Verification items for the finished model (mm, model axes). Give positions to 0.01 mm unless a question says otherwise; leave off trailing zeros. Order: outer loops, then holes, each group sorted by start corner. A loop starts at its lowest first (then second) coordinate and runs counter-clockwise, first axis right, second up. Notation, with made-up numbers: (-21, 55.25) - (17, 55.25) arc R28 ccw to (17, 78.25) - close; hole circle Ø3 at (-23.5, 14). An arc over 180 degrees is marked (long way). Answer as a JSON object with one key per item and string values. Group by question number.
(1) Mould release check, pull along Z, two halves, no side actions. Record for faces 1 (the face through (2, 7, 34.546)), 2 (the face through (-1.596, 6.902, -5.915)), 3 (the face through (2, 0, -1)), 4 (the face through (2, 7, -36.182)): +Z half, -Z half, draft (parallel to the pull), parting line (faces both ways), or undercut.
(2) Section check B-B (x = 3). Record the boundary of the cut face in (y, z).
(3) Section check C-C (y = 7). Record the boundary of the cut face in (x, z).
(4) Section check A-A (z = -17). Record the boundary of the cut face in (x, y).
(5) Thickness scan on line 1 (Z direction, x = 3, y = 6); line 2 (X direction, y = 6.25, z = -17); line 3 (Z direction, x = -7, y = 10.25). Record the ranges inside material, lowest first.
```python
from build123d import *

# Parameters (mm, degrees)
IZIM1_W                     = 46.198257095
IZIM1_H                     = 70.728305111
Y_KSEKLIK_EKSTR_ZYON1_DEPTH = 14
IZIM2_R                     = 12
KES_EKSTR_ZYON1_DEPTH       = 15


with BuildPart() as part:
    # Çizim1 → Yükseklik-Ekstrüzyon1 (new body)
    with BuildSketch(Plane(origin=(0, 0, 0), x_dir=(1, 0, 0), z_dir=(0, 1, 0))):
        with Locations((2.453004802, 0.817668268)):
            Rectangle(IZIM1_W, IZIM1_H)
    extrude(amount=Y_KSEKLIK_EKSTR_ZYON1_DEPTH)

    # Çizim2 → Kes-Ekstrüzyon1 (cut)
    with BuildSketch(Plane(origin=(0, 0, 0), x_dir=(1, 0, 0), z_dir=(0, 1, 0))):
        with Locations(Location((3, 17, 0), (0, 0, 270))):
            Circle(IZIM2_R)
    extrude(amount=KES_EKSTR_ZYON1_DEPTH, mode=Mode.SUBTRACT)


solid = part.part
```
Solutions:
{
 "1": {"face 1": "+Z half", "face 2": "undercut", "face 3": "draft", "face 4": "-Z half"},
 "2": {"outline": "(0, -36.18) - (14, -36.18) - (14, -29) - (0, -29) - close; (0, -5) - (14, -5) - (14, 34.55) - (0, 34.55) - close"},
 "3": {"outline": "(-20.65, -36.18) - (25.55, -36.18) - (25.55, 34.55) - (-20.65, 34.55) - close; hole circle Ø24 at (3, -17)"},
 "4": {"outline": "(-20.65, 0) - (-9, 0) - (-9, 14) - (-20.65, 14) - close; (15, 0) - (25.55, 0) - (25.55, 14) - (15, 14) - close"},
 "5": {"line 1": "z = -36.18 to -29, -5 to 34.55", "line 2": "x = -20.65 to -9, 15 to 25.55", "line 3": "z = -36.18 to -23.63, -10.37 to 34.55"}
}
